from build123d import *

# Parameters (mm, degrees)
SKETCH1_R           = 4
SKETCH1_R_2         = 1.75
BOSS_EXTRUDE1_DEPTH = 6
SKETCH2_R           = 12.5
SKETCH2_R_2         = 4
BOSS_EXTRUDE2_DEPTH = 13
SKETCH4_W           = 3
SKETCH4_H           = 2.4
CUT_EXTRUDE2_DEPTH  = 30
SKETCH3_R           = 1.65
CUT_EXTRUDE3_DEPTH  = 14
SKETCH5_R           = 1.65
CUT_EXTRUDE4_DEPTH  = 30
BOSS_EXTRUDE3_START = -6
BOSS_EXTRUDE3_DEPTH = 6


with BuildPart() as part:
    # Sketch1 → Boss-Extrude1 (new body)
    with BuildSketch(Plane(origin=(0, 0, 0), x_dir=(1, 0, 0), z_dir=(0, 1, 0))):
        with BuildLine():
            Line((-14.071247279, 13.5), (14.071247279, 13.5))
            ThreePointArc((14.071247279, 13.5), (19.5, 0), (14.071247279, -13.5))
            Line((14.071247279, -13.5), (-14.071247279, -13.5))
            ThreePointArc((-14.071247279, -13.5), (-19.5, 0), (-14.071247279, 13.5))
        make_face()
        with Locations(Location((0, 0, 0), (0, 0, 270))):
            Circle(SKETCH1_R, mode=Mode.SUBTRACT)
        with Locations(Location((-12.5, 10, 0), (0, 0, 270))):
            Circle(SKETCH1_R_2, mode=Mode.SUBTRACT)
        with Locations(Location((-12.5, -10, 0), (0, 0, 270))):
            Circle(SKETCH1_R_2, mode=Mode.SUBTRACT)
        with Locations(Location((12.5, -10, 0), (0, 0, 270))):
            Circle(SKETCH1_R_2, mode=Mode.SUBTRACT)
        with Locations(Location((12.5, 10, 0), (0, 0, 270))):
            Circle(SKETCH1_R_2, mode=Mode.SUBTRACT)
    extrude(amount=BOSS_EXTRUDE1_DEPTH)

    # Sketch2 → Boss-Extrude2 (add)
    with BuildSketch(Plane(origin=(0, 6, 0), x_dir=(1, 0, 0), z_dir=(0, 1, 0))):
        with Locations(Location((0, 0, 0), (0, 0, 90))):
            Circle(SKETCH2_R)
        with Locations(Location((0, 0, 0), (0, 0, 270))):
            Circle(SKETCH2_R_2, mode=Mode.SUBTRACT)
    extrude(amount=BOSS_EXTRUDE2_DEPTH)

    # Sketch4 → Cut-Extrude2 (cut)
    with BuildSketch(Plane(origin=(0, 19, 0), x_dir=(1, 0, 0), z_dir=(0, 1, 0))):
        with Locations((0, 4)):
            Rectangle(SKETCH4_W, SKETCH4_H)
    extrude(amount=-CUT_EXTRUDE2_DEPTH, mode=Mode.SUBTRACT)

    # Sketch3 → Cut-Extrude3 (cut)
    with BuildSketch(Plane(origin=(0, 0, -13.5), x_dir=(-1, 0, 0), z_dir=(0, 0, -1))):
        with Locations(Location((0, 13, 0), (0, 0, 335.380022671))):
            Circle(SKETCH3_R)
    extrude(amount=-CUT_EXTRUDE3_DEPTH, mode=Mode.SUBTRACT)

    # Sketch5 → Cut-Extrude4 (cut)
    with BuildSketch(Plane(origin=(0, 0, 0), x_dir=(0, 0, -1), z_dir=(1, 0, 0))):
        with Locations((0, 13)):
            Circle(SKETCH5_R)
    extrude(amount=-CUT_EXTRUDE4_DEPTH, mode=Mode.SUBTRACT)

    # Sketch6 → Boss-Extrude3 (add)
    with BuildSketch(Plane(origin=(0, 6, 0), x_dir=(1, 0, 0), z_dir=(0, 1, 0)).offset(BOSS_EXTRUDE3_START)):
        with BuildLine():
            Line((-14.071247279, 13.5), (14.071247279, 13.5))
            ThreePointArc((14.071247279, 13.5), (0, 19.5), (-14.071247279, 13.5))
        make_face()
        with BuildLine():
            Line((14.071247279, -13.5), (-14.071247279, -13.5))
            ThreePointArc((-14.071247279, -13.5), (0, -19.5), (14.071247279, -13.5))
        make_face()
    extrude(amount=BOSS_EXTRUDE3_DEPTH)


solid = part.part
The listing builds one solid part. Answer for the finished solid, in the listing's coordinates (mm). A direction names the side the tool comes from. Give positions to 0.01 mm unless a question says otherwise; leave off trailing zeros. Write each loop counter-clockwise with the first axis right and the second up, starting at its lowest first coordinate (ties: lowest second). Pieces come first, ordered by that corner, then holes.
Item 1: Determine the mould class of faces 1 (the flat face through (1.5, 6, -4)), 2 (the cylindrical face through (-3.755, 12.409, -11.923)), 3 (the flat face through (0, 6, 13)) for opening direction Z: released by +Z, released by -Z, zero draft, split by the parting line, or undercut.
Item 2: Section A-A, the plane z = -10 is taken. Write down the section's boundary in (x, y).
Item 3: Section C-C, the plane y = 10.25 is taken. Write down the section's boundary in (x, z).
Item 4: Flat-ended cylindrical pins translate along their axes: P1, Ø4.5, axis at x = -12.5, z = -10, coming from the +Y side; P2, Ø1.5, axis at x = 11.5, y = 6, coming from the -Z side; P3, Ø4.5, axis at x = 0, y = 13, coming from the -Z side. Find the tip coordinate at first contact, or state that the pin passes through.
Item 5: Find the intervals of material crossed by line 1 along Y through (x, z) = (-8, 10.5); line 2 along X through (y, z) = (4.75, 0); line 3 along X through (y, z) = (10, 0), in increasing order.
Item 6: Which of the six approach directions +Z, -Z, +X, -X, +Y, -Y give full straight-line access (tool end or side, diameter ignored) to faces 4 (the flat face through (-1.5, 16, -4)), 5 (the cylindrical face through (-8, 11.4, 0.4)), 6 (the cylindrical face through (-0.08, 11.35, -9.12)), 7 (the flat face through (-5, 0, 0))?
Item 7: Section D-D, the plane z = 0 is taken. Write down the section's boundary in (x, y).
Item 8: Section B-B, the plane x = 0 is taken. Write down the section's boundary in (y, z), plus the area to 3 significant figures.
Completed:
1. face 1: undercut
1. face 2: split by the parting line
1. face 3: zero draft
2. outline: (-16.74, 0) - (-14.25, 0) - (-14.25, 6) - (-16.74, 6) - close; (-10.75, 0) - (10.75, 0) - (10.75, 6) - (7.5, 6) - (7.5, 19) - (-7.5, 19) - (-7.5, 6) - (-10.75, 6) - close; (14.25, 0) - (16.74, 0) - (16.74, 6) - (14.25, 6) - close; hole circle Ø3.3 at (0, 13)
3. outline: circle Ø25 at (0, 0); hole (-1.5, -5.2) - (1.5, -5.2) - (1.5, -3.71) arc R4 ccw (long way) to (-1.5, -3.71) - close
4. P1: stops at y = 6
4. P2: stops at z = -16.27
4. P3: stops at z = -12.5
5. line 1: y = 0 to 6
5. line 2: x = -19.5 to -4, 4 to 19.5
5. line 3: x = -12.5 to -4, 4 to 12.5
6. face 4: +Y, -Y
6. face 5: -X
6. face 6: -Z
6. face 7: +Z, -Z, +X, -X, -Y
7. outline: (-19.5, 0) - (-4, 0) - (-4, 11.35) - (-12.5, 11.35) - (-12.5, 6) - (-19.5, 6) - close; (-12.5, 14.65) - (-4, 14.65) - (-4, 19) - (-12.5, 19) - close; (4, 0) - (19.5, 0) - (19.5, 6) - (12.5, 6) - (12.5, 19) - (4, 19) - close
8. outline: (0, -19.5) - (6, -19.5) - (6, -12.5) - (11.35, -12.5) - (11.35, -5.2) - (0, -5.2) - close; (0, 4) - (19, 4) - (19, 12.5) - (6, 12.5) - (6, 19.5) - (0, 19.5) - close; (14.65, -12.5) - (19, -12.5) - (19, -5.2) - (14.65, -5.2) - close
8. area: 360 mm2
